Verification items for the finished model (mm, model axes). Face numbers are marked on the shaded views. A direction names the side the tool comes from. Coordinates: 2 decimals unless noted, no trailing zeros. Answer in a Markdown table with one row per item.
```python
from build123d import *


with BuildPart() as part:
    # Sketch1 → Revolve1 (revolve)
    with BuildSketch(Plane(origin=(0, 0, 0), x_dir=(-1, 0, 0), z_dir=(0, 1, 0))):
        Polygon((-17.4625, -6.35), (-17.4625, 1.74625), (-17.350532367, 2.38125), (-19.05, 2.38125), (-19.05, 3.81), (-18.938032367, 4.445), (-12.7, 4.445), (-12.7, 6.35), (-6.35, 6.35), (-6.35, -6.35), align=None)
    revolve(axis=Axis((0, 0, 114.851664886), (0, 0, -1)))


solid = part.part
```
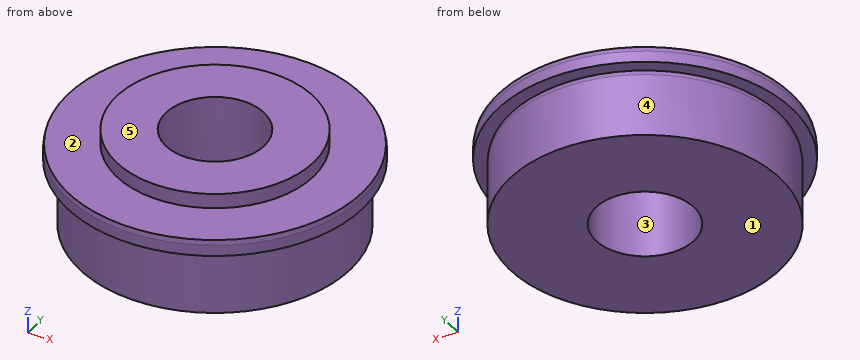
1. Material ranges on probe 1 along Y at (x, z) = (0, -3.5); probe 2 along X at (y, z) = (0, 3.75), recorded low to high. Write a range as from..to.
Findings below:
| item | result |
|---|---|
| probe 1 | y = -17.46..-6.35, 6.35..17.46 |
| probe 2 | x = -19.05..-6.35, 6.35..19.05 |
2. Release check for a two-part mould opening along X. For the marked faces 3, 4 and 5 record: released by +X, released by -X, zero draft, split by the parting line, or undercut.
Findings below:
| item | result |
|---|---|
| face 3 | undercut |
| face 4 | split by the parting line |
| face 5 | zero draft |
3. Go/stop test with flat-tipped pins: pin 1 (12 mm diameter, centred on x = -11.5, y = -15, fed in from -Z); pin 2 (5 mm diameter, centred on x = 11, z = -2.5, fed in from -Y); pin 3 (5 mm diameter, centred on x = -13, y = 11.5, fed in from +Z) (3 decimals). Record where each tip stops, or that it passes through.
Findings below:
| item | result |
|---|---|
| pin 1 | stops at z = -6.35 |
| pin 2 | stops at y = -15.25 |
| pin 3 | stops at z = 4.445 |
4. Access from +Z, -Z, +X, -X, +Y, -Y to the whole of each face (thin tool, end or side, straight path). Record for the marked faces 1 and 2.
Findings below:
| item | result |
|---|---|
| face 1 | -Z, +X, -X, +Y, -Y |
| face 2 | +Z |
